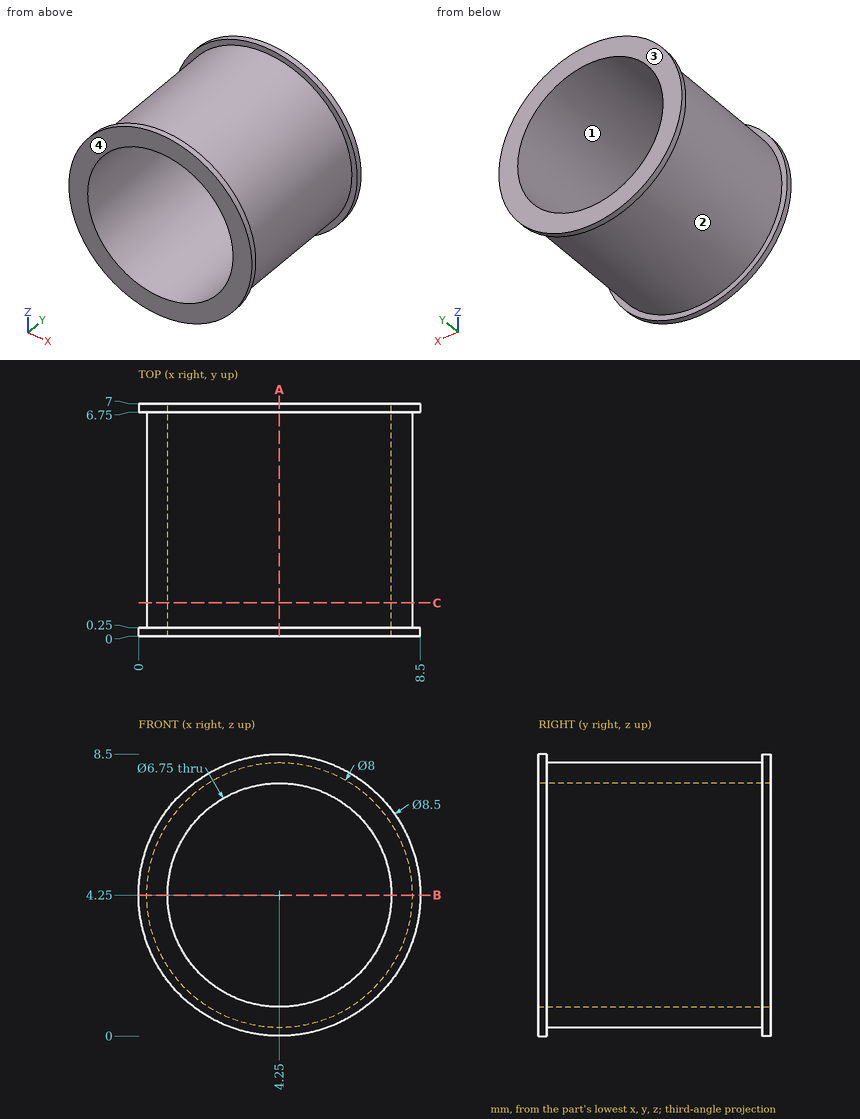
Geometry check sheet. Reference: drawing and pictorial views, mm from the part's lowest x, y, z. Give positions to 0.01 mm unless a question says otherwise; leave off trailing zeros. Loops run counter-clockwise (first coordinate to the right, second up) from the corner with the lowest first, then second, coordinate; pieces in that order, holes last.
1. Thickness scan on line 1 (X direction, y = 4, z = 4.25) (3 decimals); line 2 (Z direction, x = 5.25, y = 2). Record the ranges inside material, lowest first.
2. Section check B-B, the plane z = 4.25. Enter the section's corners in (x, y) (3 decimals).
3. Mould release check, pull along Y, two halves, no side actions. Record for the marked faces 1, 2, 3 and 4: released by +Y, released by -Y, zero draft, split by the parting line, or undercut.
4. Section check C-C, the plane y = 1. Enter the section's corners in (x, z) (3 decimals), then the cut area to 3 significant figures.
5. Go/stop test with flat-tipped pins: pin 1 Ø3 at (y, z) = (2, 4.5) entering from -X; pin 2 Ø4 at (x, z) = (4, 3.5) entering from +Y; pin 3 Ø3 at (x, y) = (4.5, 2) entering from -Z; pin 4 Ø2 at (y, z) = (3, 7) entering from +X. Record where each tip stops, or that it passes through.
6. Section check A-A, the plane x = 4.25. Enter the section's corners in (y, z) (3 decimals).
Geometry says:
1. line 1: x = 0.25 to 0.875, 7.625 to 8.25
1. line 2: z = 0.38 to 1.03, 7.47 to 8.12
2. outline: (0, 0) - (0.875, 0) - (0.875, 7) - (0, 7) - (0, 6.75) - (0.25, 6.75) - (0.25, 0.25) - (0, 0.25) - close; (7.625, 0) - (8.5, 0) - (8.5, 0.25) - (8.25, 0.25) - (8.25, 6.75) - (8.5, 6.75) - (8.5, 7) - (7.625, 7) - close
3. face 1: zero draft
3. face 2: undercut
3. face 3: released by +Y
3. face 4: released by -Y
4. outline: circle Ø8 at (4.25, 4.25); hole circle Ø6.75 at (4.25, 4.25)
4. area: 14.5 mm2
5. pin 1: stops at x = 0.25
5. pin 2: passes through
5. pin 3: stops at z = 0.25
5. pin 4: stops at x = 7.85
6. outline: (0, 0) - (0.25, 0) - (0.25, 0.25) - (6.75, 0.25) - (6.75, 0) - (7, 0) - (7, 0.875) - (0, 0.875) - close; (0, 7.625) - (7, 7.625) - (7, 8.5) - (6.75, 8.5) - (6.75, 8.25) - (0.25, 8.25) - (0.25, 8.5) - (0, 8.5) - close
